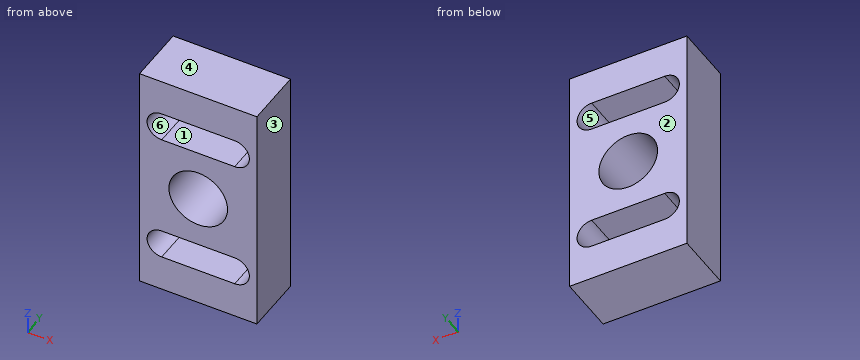
```python
from build123d import *

# Parameters (mm, degrees)
SKETCH1_W           = 12.7
SKETCH1_H           = 25.4
BOSS_EXTRUDE1_DEPTH = 6.35
SKETCH2_R           = 3.175
CUT_EXTRUDE1_DEPTH  = 16.554259867
CUT_EXTRUDE2_DEPTH  = 16.554259867


with BuildPart() as part:
    # Sketch1 → Boss-Extrude1 (new body)
    with BuildSketch(Plane(origin=(0, 0, 0), x_dir=(1, 0, 0), z_dir=(0, 1, 0))):
        Rectangle(SKETCH1_W, SKETCH1_H)
    extrude(amount=BOSS_EXTRUDE1_DEPTH)

    # Sketch2 → Cut-Extrude1 (cut, through all)
    with BuildSketch(Plane(origin=(0, 6.35, 0), x_dir=(1, 0, 0), z_dir=(0, 1, 0))):
        with Locations(Location((0, 0, 0), (0, 0, 270))):
            Circle(SKETCH2_R)
    extrude(amount=-CUT_EXTRUDE1_DEPTH, mode=Mode.SUBTRACT)

    # Sketch3 → Cut-Extrude2 (cut, through all)
    with BuildSketch(Plane(origin=(0, 6.35, 0), x_dir=(1, 0, 0), z_dir=(0, 1, 0))):
        with BuildLine():
            Line((-3.949618405, 8.764602641), (3.949618405, 8.764602641))
            ThreePointArc((3.949618405, 8.764602641), (5.537118405, 7.177102641), (3.949618405, 5.589602641))
            Line((3.949618405, 5.589602641), (-3.949618405, 5.589602641))
            ThreePointArc((-3.949618405, 5.589602641), (-5.537118405, 7.177102641), (-3.949618405, 8.764602641))
        make_face()
    cut_extrude2 = extrude(amount=-CUT_EXTRUDE2_DEPTH, mode=Mode.SUBTRACT)

    # Mirror1: Cut-Extrude2 across plane
    add(cut_extrude2.mirror(Plane.XY), mode=Mode.SUBTRACT)


solid = part.part
```
Geometry check sheet. Reference: the model listing, model coordinates, mm. Face numbers are marked on the shaded views. A direction names the side the tool comes from. Round coordinates to 2 decimals unless told otherwise and drop trailing zeros. Loops run counter-clockwise (first coordinate to the right, second up) from the corner with the lowest first, then second, coordinate; pieces in that order, holes last. Notation, with made-up numbers: (12.25, 60) - (17.25, 60) arc R33 ccw to (17.25, 91) - close; hole circle Ø1 at (-28.75, 79). An arc over 180 degrees is marked (long way). Use a Markdown table: item, result.
Q1. Access from +Z, -Z, +X, -X, +Y, -Y to the whole of each face (thin tool, end or side, straight path). Record for the marked faces 1 and 2.
Solutions:
| item | result |
|---|---|
| face 1 | +Y, -Y |
| face 2 | +Z, -Z, +X, -X, +Y |
Q2. Draft check along X on the marked faces 3, 4, 5 and 6. Enter one of: released by +X, released by -X, zero draft, split by the parting line, or undercut.
Solutions:
| item | result |
|---|---|
| face 3 | released by +X |
| face 4 | zero draft |
| face 5 | undercut |
| face 6 | undercut |
Q3. Cross-section at C-C on y = 5. State how many separate pieces and enclosed holes the cut face has, plus the area to 3 significant figures.
Solutions:
| item | result |
|---|---|
| separate pieces | 1 |
| enclosed holes | 3 |
| area | 225 mm2 |
Q4. Material ranges on line 1 (Z direction, x = 3.25, y = 4); line 2 (Z direction, x = -5, y = 1.5); line 3 (Z direction, x = 0.5, y = 3), recorded low to high.
Solutions:
| item | result |
|---|---|
| line 1 | z = -12.7 to -8.76, -5.59 to 5.59, 8.76 to 12.7 |
| line 2 | z = -12.7 to -8.37, -5.99 to 5.99, 8.37 to 12.7 |
| line 3 | z = -12.7 to -8.76, -5.59 to -3.14, 3.14 to 5.59, 8.76 to 12.7 |
Q5. Cross-section at D-D on x = 0. Record the cut outline in (y, z) (3 decimals).
Solutions:
| item | result |
|---|---|
| outline | (0, -12.7) - (6.35, -12.7) - (6.35, -8.765) - (0, -8.765) - close; (0, -5.59) - (6.35, -5.59) - (6.35, -3.175) - (0, -3.175) - close; (0, 3.175) - (6.35, 3.175) - (6.35, 5.59) - (0, 5.59) - close; (0, 8.765) - (6.35, 8.765) - (6.35, 12.7) - (0, 12.7) - close |
Q6. Cross-section at B-B on x = -3.5. Record the cut outline in (y, z).
Solutions:
| item | result |
|---|---|
| outline | (0, -12.7) - (6.35, -12.7) - (6.35, -8.76) - (0, -8.76) - close; (0, -5.59) - (6.35, -5.59) - (6.35, 5.59) - (0, 5.59) - close; (0, 8.76) - (6.35, 8.76) - (6.35, 12.7) - (0, 12.7) - close |
Q7. Cross-section at A-A on z = 0. Record the cut outline in (x, y) (3 decimals), plus the area to 3 significant figures.
Solutions:
| item | result |
|---|---|
| outline | (-6.35, 0) - (-3.175, 0) - (-3.175, 6.35) - (-6.35, 6.35) - close; (3.175, 0) - (6.35, 0) - (6.35, 6.35) - (3.175, 6.35) - close |
| area | 40.3 mm2 |
